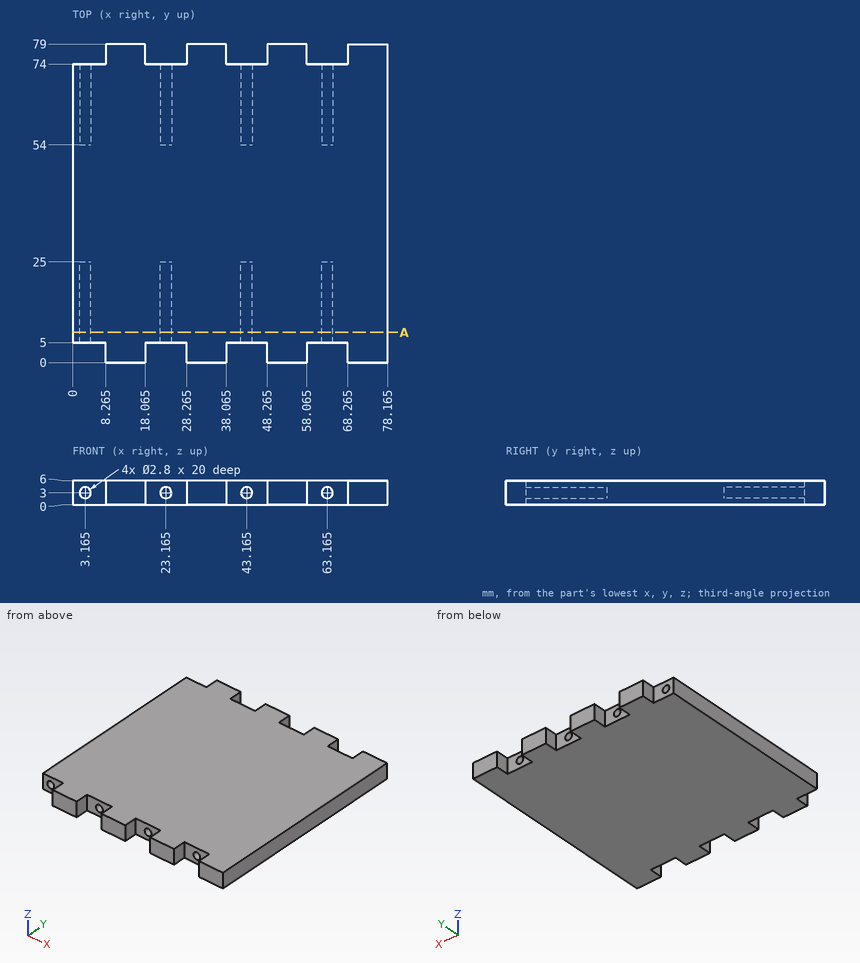
Input: dimensioned drawing with shaded views. Units: mm. Origin: part minimum x, y, z. Coordinates: 2 decimals unless noted, no trailing zeros. Loops run counter-clockwise (first coordinate to the right, second up) from the corner with the lowest first, then second, coordinate; pieces in that order, holes last. Notation, with made-up numbers: M 71.5,82 L 92.5,82 A13 cw 92.5,91 Z; hole C 38.5,80 d10. An arc over 180 degrees is marked long. One line per item, written item: value.
(1) Pin query (flat end, axial travel): pin 1 (3 mm diameter, centred on x = 23, z = 2.5, fed in from +Y); pin 2 (1.5 mm diameter, centred on x = 39, z = 1.5, fed in from -Y); pin 3 (1.5 mm diameter, centred on y = 2.5, z = 3.5, fed in from -X) (1 decimal). Return the tip coordinate at first contact, or that it passes through.
Filled in:
pin 1: y = 74
pin 2: y = 5
pin 3: x = 8.3
(2) Section A-A (y = 7.5). Output: boundary loops of the cut face in (x, z) (1 decimal).
Filled in:
outline: M 0,0 L 78.2,0 L 78.2,6 L 0,6 Z; hole C 3.2,3 d2.8; hole C 23.2,3 d2.8; hole C 43.2,3 d2.8; hole C 63.2,3 d2.8
(3) Line query: line 1 along X through (y, z) = (75.5, 1.95) (1 decimal); line 2 along X through (y, z) = (69, 3) (1 decimal); line 3 along X through (y, z) = (64.5, 2.15) (1 decimal). Output: solid intervals per line, ascending. Write a range as from..to.
Filled in:
line 1: 8.3..18.1, 28.3..38.1, 48.3..58.1, 68.3..78.2
line 2: 0..1.8, 4.6..21.8, 24.6..41.8, 44.6..61.8, 64.6..78.2
line 3: 0..2.1, 4.3..22.1, 24.3..42.1, 44.3..62.1, 64.3..78.2
